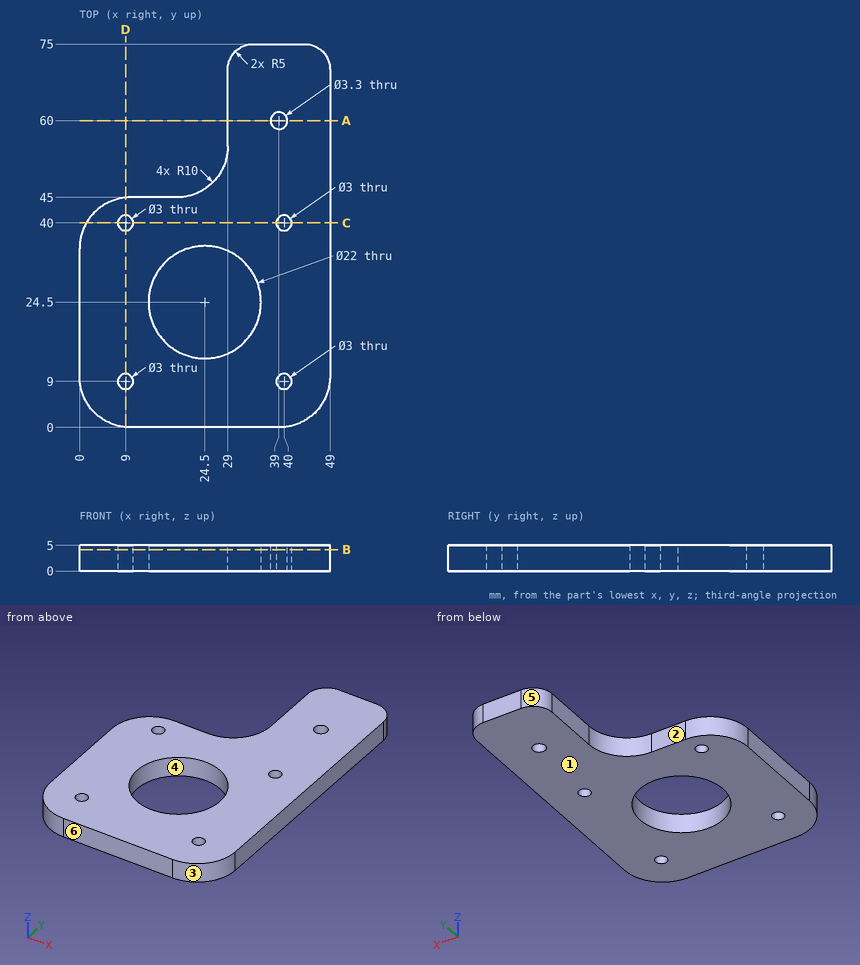
Geometry: see drawing. Coordinates: mm, zero at the bounding-box minimum. A direction names the side the tool comes from. Round coordinates to 2 decimals unless told otherwise and drop trailing zeros. Loops run counter-clockwise (first coordinate to the right, second up) from the corner with the lowest first, then second, coordinate; pieces in that order, holes last. Notation, with made-up numbers: M 51,-33.75 L 90,-33.75 A18 cw 90,-21.75 Z; hole C 0.5,-23 d1. An arc over 180 degrees is marked long. Use a Markdown table: item, result. Add a question column.
1. Cut plane A-A, the plane y = 60. Output: boundary loops of the cut face in (x, z), and give its area (3 significant figures).
2. Cut plane B-B, the plane z = 4.2. Output: boundary loops of the cut face in (x, y), and give its area (3 significant figures).
3. Contact query for flat-ended pins moving along their axis: pin 1 (3.5 mm diameter, centred on x = 9, y = 40, fed in from -Z); pin 2 (1.5 mm diameter, centred on y = 64, z = 1.5, fed in from -X); pin 3 (1.5 mm diameter, centred on x = 33, z = 1, fed in from +Y); pin 4 (1.5 mm diameter, centred on x = 24.5, z = 0.5, fed in from +Y). Output: stop coordinate, or through.
4. Pull-direction query (X, two-part tool) for the marked faces 3, 4, 5 and 6; classes: +X half, -X half, draft (parallel to the pull), parting line (faces both ways), or undercut.
5. Ray query, line 1 along Y through (x, z) = (9, 1.4); line 2 along Y through (x, z) = (40, 2.95); line 3 along X through (y, z) = (34.5, 0.6). Return the intervals inside material, ascending. Write a range as [from, to].
6. Set-up query: the marked faces 1 and 2. Return all of +Z, -Z, +X, -X, +Y, -Y with unobstructed straight access to the full face (end or side cutting, diameter ignored); none if empty.
7. Cut plane C-C, the plane y = 40. Output: boundary loops of the cut face in (x, z).
8. Cut plane D-D, the plane x = 9. Output: boundary loops of the cut face in (y, z), and give its area (3 significant figures).
Solution:
| question | item | result |
|---|---|---|
| 1 | outline | M 29,0 L 37.35,0 L 37.35,5 L 29,5 Z; M 40.65,0 L 49,0 L 49,5 L 40.65,5 Z |
| 1 | area | 83.5 mm2 |
| 2 | outline | M 0,10 A10 ccw 10,0 L 39,0 A10 ccw 49,10 L 49,70 A5 ccw 44,75 L 34,75 A5 ccw 29,70 L 29,55 A10 cw 19,45 L 10,45 A10 ccw 0,35 Z; hole C 9,9 d3; hole C 9,40 d3; hole C 24.5,24.5 d22; hole C 39,60 d3.3; hole C 40,9 d3; hole C 40,40 d3 |
| 2 | area | 2,330 mm2 |
| 3 | pin 1 | stops at z = 0 |
| 3 | pin 2 | stops at x = 29 |
| 3 | pin 3 | stops at y = 74.99 |
| 3 | pin 4 | stops at y = 47.19 |
| 4 | face 3 | +X half |
| 4 | face 4 | undercut |
| 4 | face 5 | -X half |
| 4 | face 6 | draft |
| 5 | line 1 | y = [0.05, 7.5], [10.5, 38.5], [41.5, 44.95] |
| 5 | line 2 | y = [0.05, 7.5], [10.5, 38.5], [41.5, 58.69], [61.31, 75] |
| 5 | line 3 | x = [0, 19.92], [29.08, 49] |
| 6 | face 1 | -Z, +X, -X, +Y, -Y |
| 6 | face 2 | +Z, -Z, -X, +Y |
| 7 | outline | M 1.34,0 L 7.5,0 L 7.5,5 L 1.34,5 Z; M 10.5,0 L 38.5,0 L 38.5,5 L 10.5,5 Z; M 41.5,0 L 49,0 L 49,5 L 41.5,5 Z |
| 8 | outline | M 0.05,0 L 7.5,0 L 7.5,5 L 0.05,5 Z; M 10.5,0 L 38.5,0 L 38.5,5 L 10.5,5 Z; M 41.5,0 L 44.95,0 L 44.95,5 L 41.5,5 Z |
| 8 | area | 194 mm2 |
